Source: CAD feature listing. Evaluate the final solid. Frame: model axes, mm. Face numbers are marked on the shaded views. A direction names the side the tool comes from. Coordinates: 2 decimals unless noted, no trailing zeros. Write each loop counter-clockwise with the first axis right and the second up, starting at its lowest first coordinate (ties: lowest second). Pieces come first, ordered by that corner, then holes. Notation, with made-up numbers: (-10, 41.5) -> (5, 41.5) arc R19 cw to (5, 73.5) -> close; hole circle Ø9 at (-6, 18). An arc over 180 degrees is marked (long way). Write item = value, one per line.
Autodesk Inventor part; units mm, degrees
ref_plane "YZ Plane" through (0, 0, 0) normal (1, 0, 0) x (0, 1, 0)
ref_plane "XZ Plane" through (0, 0, 0) normal (0, 1, 0) x (-1, 0, 0)
ref_plane "XY Plane" through (0, 0, 0) normal (0, 0, 1) x (1, 0, 0)
sketch "Sketch3" plane through (0, 0, 0) normal (0, 1, 0) x (-1, 0, 0)
  line L0 (-8, 16) -> (8, 16)
  line L1 (8, 16) -> (8, -16)
  line L2 (8, -16) -> (-8, -16)
  line L3 (-8, -16) -> (-8, 16)
  line L4 (-8, 16) -> (8, -16) construction
  line L5 (8, 16) -> (-8, -16) construction
  point P0 (0, 0)
  dimension "d7" = 16
  dimension "d8" = 32
extrude "Extrusion1" add sketch "Sketch3" along normal blind 4.5
sketch "Sketch4" plane through (0, 0, 0) normal (0, -1, 0) x (1, 0, 0)
  line L0 (0, 0) -> (0, 9)
  line L1 (0, 9) -> (0, -9)
  line L2 (8, 16) -> (8, -16)
  line L3 (-8, -9) -> (8, -9)
  line L4 (8, -9) -> (8, 9)
  line L5 (8, 9) -> (-8, 9)
  line L6 (-8, 9) -> (-8, -9)
  line L7 (-8, -9) -> (8, 9) construction
  line L8 (8, -9) -> (-8, 9) construction
  dimension "d11" = 9
  dimension "d12" = 18
  dimension "d13" = 41.633
extrude "Extrusion2" add sketch "Sketch4" along normal blind 0.5
chamfer "Chamfer1" distance 0.5 angle 45 1 edges at (0, -0.5, 9)
chamfer "Chamfer2" distance 0.5 angle 45 1 edges at (0, -0.5, -9)
sketch "Sketch5" plane through (0, 4.5, 0) normal (0, 1, 0) x (1, 0, 0)
  line L0 (8, -16) -> (8, 16)
  line L1 (-8, -9) -> (8, -9)
  line L2 (8, -9) -> (8, 9)
  line L3 (8, 9) -> (-8, 9)
  line L4 (-8, 9) -> (-8, -9)
  line L5 (-8, -9) -> (8, 9) construction
  line L6 (8, -9) -> (-8, 9) construction
  point P0 (0, 0)
  dimension "d22" = 18
extrude "Extrusion3" add sketch "Sketch5" along normal blind 3
chamfer "Chamfer3" distance 2 angle 45 2 edges at (0, 7.5, 9) (0, 7.5, -9)
sketch "Sketch6" plane through (0, 4.5, 0) normal (0, 1, 0) x (1, 0, 0)
  line L0 (-8, -9) -> (-8, -16) construction
  line L1 (-8, -12.5) -> (8, -12.5) construction
  line L2 (8, -9) -> (8, -16) construction
  circle A0 centre (4, -12.5) radius 3 construction
  line L3 (8, -16) -> (-8, -16) construction
  line L4 (0, -16) -> (0, 17.9963) construction
  circle A1 centre (-4, -12.5) radius 3 construction
  line L5 (-8, -8.5) -> (-8, 8.5) construction
  line L6 (-8, 0) -> (8, 0) construction
  line L7 (8, 8.5) -> (8, -8.5) construction
  circle A2 centre (4, 12.5) radius 3 construction
  circle A3 centre (-4, 12.5) radius 3 construction
  circle A4 centre (4, -12.5) radius 3
  circle A5 centre (-4, -12.5) radius 3 construction
  circle A6 centre (-4, -12.5) radius 3
  circle A7 centre (4, 12.5) radius 3 construction
  circle A8 centre (-4, 12.5) radius 3 construction
  circle A9 centre (4, 12.5) radius 3
  circle A10 centre (-4, 12.5) radius 3 construction
  circle A11 centre (-4, 12.5) radius 3
  point P0 (0, 0)
  dimension "d28" = 6
  dimension "d29" = 4
  dimension "d30" = 33.9963
extrude "Extrusion4" cut sketch "Sketch6" against normal blind 3
sketch "Sketch7" plane through (0, 4.5, 0) normal (0, 1, 0) x (1, 0, 0)
  circle A0 centre (-4, -12.5) radius 3 construction
  line L0 (-7, -12.5) -> (-4, -12.5) construction
  circle A1 centre (4, -12.5) radius 3 construction
  line L1 (-4, -12.5) -> (4, -12.5) construction
  circle A2 centre (4, 12.5) radius 3 construction
  line L2 (4, -12.5) -> (4, 12.5) construction
  circle A3 centre (-4, 12.5) radius 3 construction
  line L3 (4, 12.5) -> (-4, 12.5) construction
  circle A4 centre (-4, -12.5) radius 1.75
  circle A5 centre (4, -12.5) radius 1.75
  circle A6 centre (4, 12.5) radius 1.75
  circle A7 centre (-4, 12.5) radius 1.75
  point P0 (0, 0)
  dimension "d33" = 3.5
  dimension "d34" = 3.5
  dimension "d35" = 3.5
  dimension "d36" = 3.5
extrude "Extrusion5" cut sketch "Sketch7" against normal blind 5
sketch "Sketch8" plane through (0, 7.5, 0) normal (0, 1, 0) x (1, 0, 0)
  circle A0 centre (0, 0) radius 1.5
  dimension "d39" = 3
extrude "Extrusion6" cut sketch "Sketch8" against normal blind 99
chamfer "Chamfer4" distance 1 angle 45 1 edges at (-1.5, 7.5, 0)
sketch "Sketch9" plane through (8, 0, 16) normal (1, 0, 0) x (0, 0, -1)
  line L0 (17.5, -0.5) -> (14.5, -0.5)
  circle A0 centre (16, -0.5) radius 4
  point P0 (16, 0)
  dimension "d45" = 8
extrude "Extrusion7" cut sketch "Sketch9" against normal blind 99
properties part number "Upper Base Bearing Holder" material "Brass, Soft Yellow"
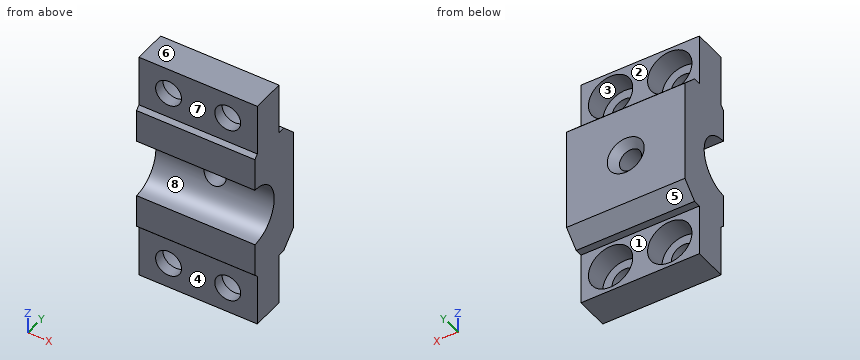
1) Pull-direction query (Z, two-part tool) for the marked faces 5, 6, 7 and 8; classes: +Z half, -Z half, draft (parallel to the pull), parting line (faces both ways), or undercut.
Answer block:
face_5 = -Z half
face_6 = +Z half
face_7 = draft
face_8 = undercut
2) First-contact query: pin 1 Ø5 at (x, z) = (-4, -12.5) entering from +Y; pin 2 Ø5.5 at (x, z) = (-0.5, 12) entering from -Y; pin 3 Ø5 at (x, z) = (-3.5, 12) entering from +Y; pin 4 Ø8 at (x, z) = (-4.5, 1.5) entering from -Y. Flat tips, straight axial feed; report the tip coordinate or a pass-through.
Answer block:
pin_1 = 1.5
pin_2 = 0
pin_3 = 4.5
pin_4 = -0.5
3) Cut plane C-C, the plane y = 2.5. Output: boundary loops of the cut face in (x, z), and give its area (3 significant figures).
Answer block:
outline = (-8, -16) -> (8, -16) -> (8, -2.65) -> (-8, -2.65) -> close; (-8, 2.65) -> (8, 2.65) -> (8, 16) -> (-8, 16) -> close; hole circle Ø6 at (-4, -12.5); hole circle Ø6 at (-4, 12.5); hole circle Ø6 at (4, -12.5); hole circle Ø6 at (4, 12.5)
area = 314 mm2
4) Cut plane A-A, the plane z = 0. Output: boundary loops of the cut face in (x, y).
Answer block:
outline = (-8, 3.5) -> (-1.5, 3.5) -> (-1.5, 6.5) -> (-2.5, 7.5) -> (-8, 7.5) -> close; (1.5, 3.5) -> (8, 3.5) -> (8, 7.5) -> (2.5, 7.5) -> (1.5, 6.5) -> close
5) Material intervals for probe 1 along X at (y, z) = (3.2, -12.5); probe 2 along X at (y, z) = (1.25, -12.5); probe 3 along X at (y, z) = (4.7, 0), sorted ascending. Write a range as [from, to].
Answer block:
probe_1 = [-8, -7], [-1, 1], [7, 8]
probe_2 = [-8, -5.75], [-2.25, 2.25], [5.75, 8]
probe_3 = [-8, -1.5], [1.5, 8]
6) Cut plane B-B, the plane x = 4. Give the number of separate pieces and of enclosed holes in the cut face, and give its area (3 significant figures).
Answer block:
separate_pieces = 3
enclosed_holes = 0
area = 131 mm2
7) Reachability of the marked faces 1, 2, 3 and 4 from +Z, -Z, +X, -X, +Y, -Y: full face, straight path, thin tool, end or side. Return the list, or none.
Answer block:
face_1 = -Z, +X, -X, +Y
face_2 = +Z, +X, -X, +Y
face_3 = +Y
face_4 = -Z, +X, -X, -Y
